Check sheet for the drawn part. Datum: minimum x, y, z corner. Units: mm. Coordinates: 2 decimals unless noted, no trailing zeros. Order: outer loops, then holes, each group sorted by start corner. A loop starts at its lowest first (then second) coordinate and runs counter-clockwise, first axis right, second up. Notation, with made-up numbers: (-33, 47) - (-23, 47) arc R16 ccw to (-23, 60) - close; hole circle Ø2 at (34, 44.25). An arc over 180 degrees is marked (long way). Put each result on its own line as item: value.
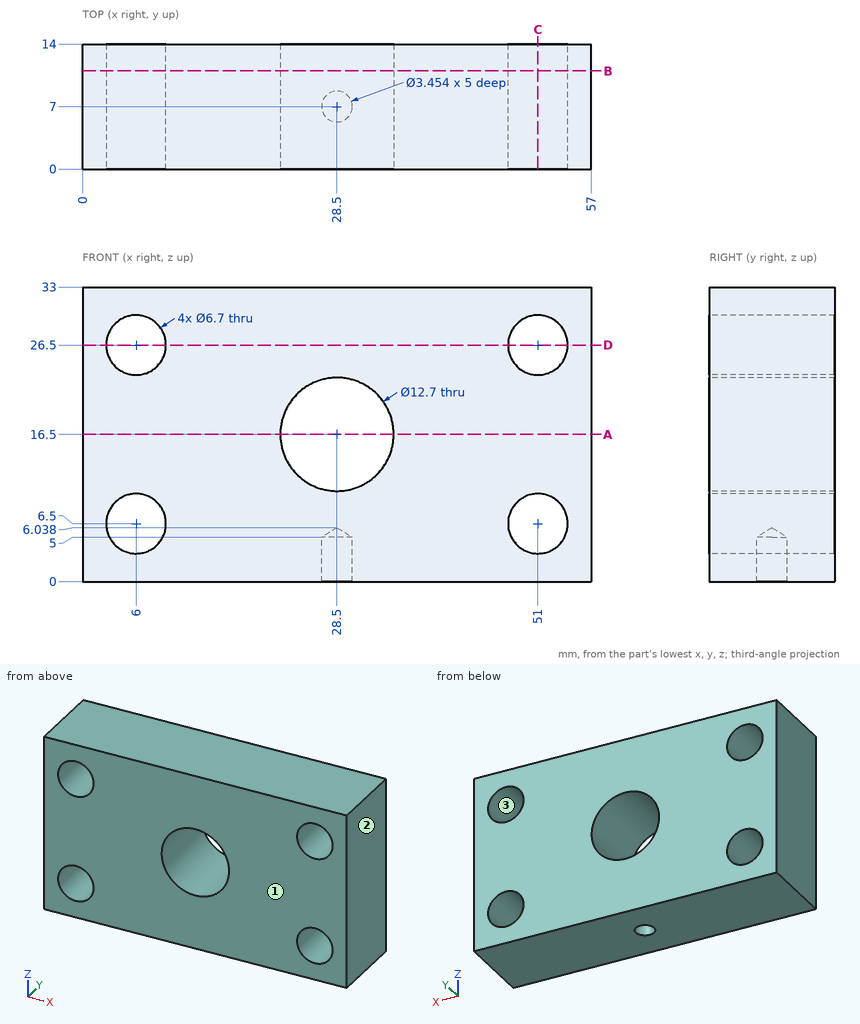
Q1. Thickness scan on L1, parallel to Z at x = 6, y = 1.5; L2, parallel to X at y = 7, z = 1.5; L3, parallel to Z at x = 50, y = 13.25. Record the ranges inside material, lowest first. Write a range as [from, to].
Answer block:
L1: z = [0, 3.15], [9.85, 23.15], [29.85, 33]
L2: x = [0, 26.77], [30.23, 57]
L3: z = [0, 3.3], [9.7, 23.3], [29.7, 33]
Q2. Section check D-D on z = 26.5. Record the boundary of the cut face in (x, y).
Answer block:
outline: (0, 0) - (2.65, 0) - (2.65, 14) - (0, 14) - close; (9.35, 0) - (47.65, 0) - (47.65, 14) - (9.35, 14) - close; (54.35, 0) - (57, 0) - (57, 14) - (54.35, 14) - close
Q3. Section check B-B on y = 11. Record the boundary of the cut face in (x, z), then the cut area to 3 significant figures.
Answer block:
outline: (0, 0) - (57, 0) - (57, 33) - (0, 33) - close; hole circle Ø6.7 at (6, 6.5); hole circle Ø6.7 at (6, 26.5); hole circle Ø12.7 at (28.5, 16.5); hole circle Ø6.7 at (51, 6.5); hole circle Ø6.7 at (51, 26.5)
area: 1,610 mm^2
Q4. Section check A-A on z = 16.5. Record the boundary of the cut face in (x, y).
Answer block:
outline: (0, 0) - (22.15, 0) - (22.15, 14) - (0, 14) - close; (34.85, 0) - (57, 0) - (57, 14) - (34.85, 14) - close
Q5. Section check C-C on x = 51. Record the boundary of the cut face in (y, z).
Answer block:
outline: (0, 0) - (14, 0) - (14, 3.15) - (0, 3.15) - close; (0, 9.85) - (14, 9.85) - (14, 23.15) - (0, 23.15) - close; (0, 29.85) - (14, 29.85) - (14, 33) - (0, 33) - close
Q6. Draft check along X on the marked faces 1, 2 and 3. Enter one of: pulls with the +X half, pulls with the -X half, needs draft (parallel to the pull), parting line crosses it, or undercut.
Answer block:
face 1: needs draft
face 2: pulls with the +X half
face 3: undercut
